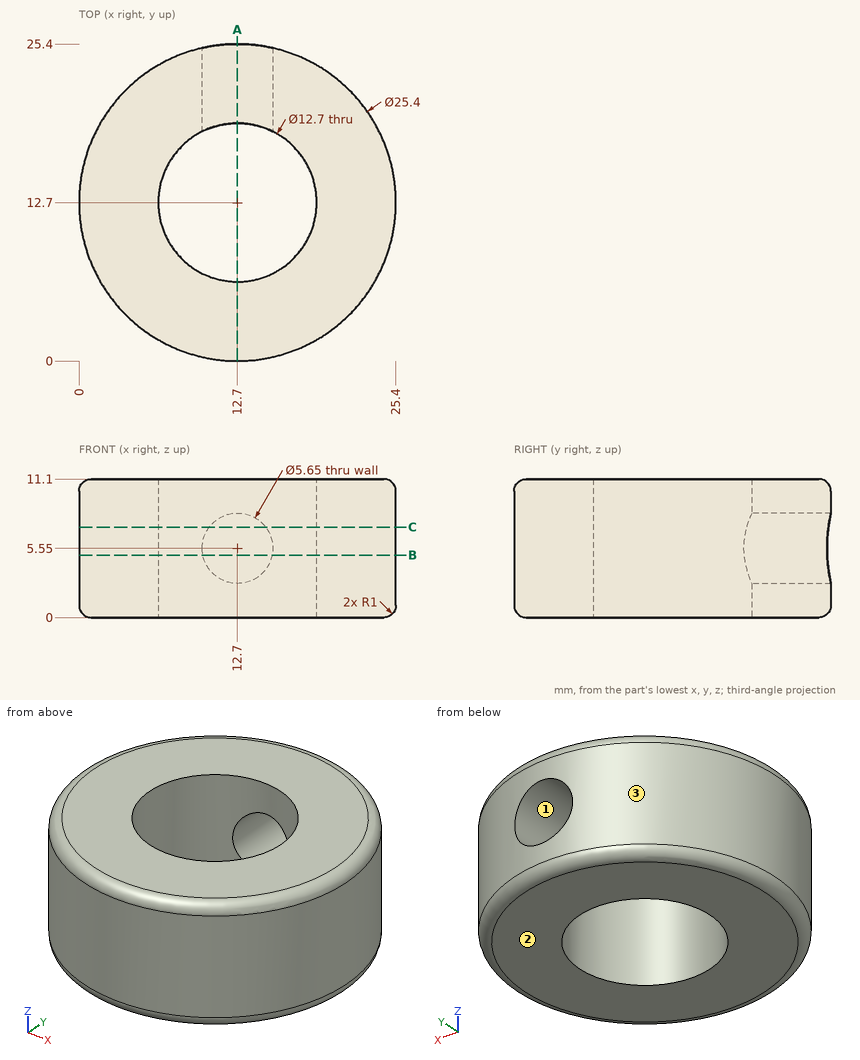
Verification items for this drawing (mm, ordinates from the low corner). Give positions to 0.01 mm unless a question says otherwise; leave off trailing zeros. Write each loop counter-clockwise with the first axis right and the second up, starting at its lowest first coordinate (ties: lowest second). Pieces come first, ordered by that corner, then holes.
1) Gauge pin test, flat ends, axial feed: pin 1 (11.5 mm diameter, centred on x = 12.7, y = 12.7, fed in from -Z); pin 2 (1 mm diameter, centred on x = 9, z = 8, fed in from +Y); pin 3 (3.5 mm diameter, centred on x = 12.7, z = 5.55, fed in from +Y). Record the tip position at first contact, or that the pin passes through.
2) Section check C-C, the plane z = 7.25. Record the boundary of the cut face in (x, y).
3) Material ranges on L1, parallel to X at y = 12.5, z = 7; L2, parallel to Z at x = 12.7, y = 21.5 (3 decimals), recorded low to high.
4) Section check B-B, the plane z = 5. Record the boundary of the cut face in (x, y).
5) Release check for a two-part mould opening along X. For the marked faces 1, 2 and 3 record: pulls with the +X half, pulls with the -X half, needs draft (parallel to the pull), parting line crosses it, or undercut.
6) Section check A-A, the plane x = 12.7. State how many separate pieces and enclosed holes the cut face has, and give its area (3 significant figures).
Computed:
1. pin 1: passes through
1. pin 2: stops at y = 24.99
1. pin 3: stops at y = 6.6
2. outline: (10.44, 18.64) - (10.44, 25.2) arc R12.7 ccw (long way) to (14.96, 25.2) - (14.96, 18.64) arc R6.35 cw (long way) to start
3. L1: x = 0 to 6.35, 19.05 to 25.4
3. L2: z = 0 to 2.725, 8.375 to 11.1
4. outline: (9.93, 18.41) - (9.93, 25.09) arc R12.7 ccw (long way) to (15.47, 25.09) - (15.47, 18.41) arc R6.35 cw (long way) to start
5. face 1: undercut
5. face 2: needs draft
5. face 3: parting line crosses it
6. separate pieces: 3
6. enclosed holes: 0
6. area: 104 mm2
